Build history of the part. All positions in model axes, mm. Face numbers are marked on the shaded views. A direction names the side the tool comes from. Give positions to 0.01 mm unless a question says otherwise; leave off trailing zeros. Order: outer loops, then holes, each group sorted by start corner. A loop starts at its lowest first (then second) coordinate and runs counter-clockwise, first axis right, second up. Notation, with made-up numbers: (-3.75, 9.5) - (9.25, 9.5) arc R18 cw to (9.25, 16.5) - close; hole circle Ø10 at (35, 4). An arc over 180 degrees is marked (long way). Answer in a Markdown table with one row per item.
```python
from build123d import *

# Parameters (mm, degrees)
F1_DEPTH = 25.4
F5_DEPTH = 19.05


# Not quite as in the source:
# - a feature of the source that left no trace in its solid (it failed there, or was rolled back) is left out


with BuildPart() as f1:
    # F0 (on Front) → F1 (new body)
    with BuildSketch(Plane.XZ):
        Polygon((0, 31.75), (0, 0), (44.45, 0), (19.05, 31.75), align=None)
    extrude(amount=F1_DEPTH)

    # F4 (on face) → F5 (join)
    with BuildSketch(Plane(origin=(0, 0, 0), x_dir=(-1, 0, 0), z_dir=(0, 1, 0))):
        Polygon((-44.45, 19.05), (-44.45, 0), (-29.21, 19.05), align=None)
    extrude(amount=-F5_DEPTH)


solid = f1.part
```
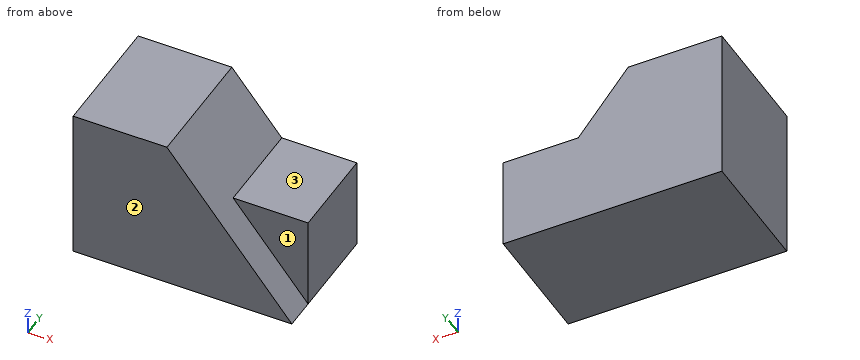
1. Probe line 1 (Z direction, x = 36, y = -16.25); line 2 (Y direction, x = 30.5, z = 18.5); line 3 (X direction, y = -19.75, z = 17.5). List the from-to ranges inside material, lowest first.
Check result:
| item | result |
|---|---|
| line 1 | z = 0 to 19.05 |
| line 2 | y = -19.05 to 0 |
| line 3 | x = 0 to 30.45 |
2. Cut at C-C on z = 28. Write the cut outline in (x, y).
Check result:
| item | result |
|---|---|
| outline | (0, -25.4) - (22.05, -25.4) - (22.05, 0) - (0, 0) - close |
3. Drop flat-ended pins along their axis: P1, Ø3, axis at y = -11.5, z = 22, coming from the +X side; P2, Ø12, axis at x = 36.5, y = -14, coming from the +Z side; P3, Ø8, axis at x = 35, z = 24, coming from the -Y side. Give the stop position or say it passes through.
Check result:
| item | result |
|---|---|
| P1 | stops at x = 28.05 |
| P2 | stops at z = 19.05 |
| P3 | passes through |
4. Cut at D-D on x = 21. Write the cut outline in (y, z), and give its area (3 significant figures).
Check result:
| item | result |
|---|---|
| outline | (-25.4, 0) - (0, 0) - (0, 29.31) - (-25.4, 29.31) - close |
| area | 745 mm² |
5. Cut at A-A on z = 6.5. Write the cut outline in (x, y), and give its area (3 significant figures).
Check result:
| item | result |
|---|---|
| outline | (0, -25.4) - (39.25, -25.4) - (39.25, -19.05) - (44.45, -19.05) - (44.45, 0) - (0, 0) - close |
| area | 1,100 mm² |
6. Which spindle directions (+Z, -Z, +X, -X, +Y, -Y) get a long thin tool onto all of the face, cutting with end or side? Do the marked faces 1, 2 and 3. Say none if no direction does.
Check result:
| item | result |
|---|---|
| face 1 | +Z, +X, -Y |
| face 2 | +Z, -Z, +X, -X, -Y |
| face 3 | +Z, +X, +Y, -Y |
7. Cut at B-B on y = -9.25. Write the cut outline in (x, z), and give its area (3 significant figures).
Check result:
| item | result |
|---|---|
| outline | (0, 0) - (44.45, 0) - (44.45, 19.05) - (29.21, 19.05) - (19.05, 31.75) - (0, 31.75) - close |
| area | 1,150 mm² |
